```python
from build123d import *

# Parameters (mm, degrees)
F0_W     = 10
F0_H     = 45
F0_R     = 1.75
F1_DEPTH = 2
F2_W     = 4
F2_H     = 10
F3_DEPTH = 10
F4_R     = 3
F5_R     = 2.5
F6_DEPTH = 25.4


with BuildPart() as f1:
    # F0 (on Top) → F1 (new body)
    with BuildSketch(Plane.XY):
        with Locations((5, 22.5)):
            Rectangle(F0_W, F0_H)
        with Locations((5, 42.5)):
            Circle(F0_R, mode=Mode.SUBTRACT)
    extrude(amount=F1_DEPTH)

    # F2 (on face) → F3 (join)
    with BuildSketch(Plane.XY.offset(2)):
        with Locations((2, 5)):
            Rectangle(F2_W, F2_H)
    extrude(amount=F3_DEPTH)

    # F4
    f4_edges = [f1.edges().sort_by_distance(p)[0] for p in [
        (10, 45, 1),
        (10, 0, 1),
        (0, 45, 1),
        (2, 0, 12),
        (2, 10, 12),
    ]]
    fillet(f4_edges, radius=F4_R)

    # F5 (on face) → F6 (cut)
    with BuildSketch(Plane.YZ.offset(4)):
        with Locations((5, 8)):
            Circle(F5_R)
    extrude(amount=-F6_DEPTH, mode=Mode.SUBTRACT)


solid = f1.part
```
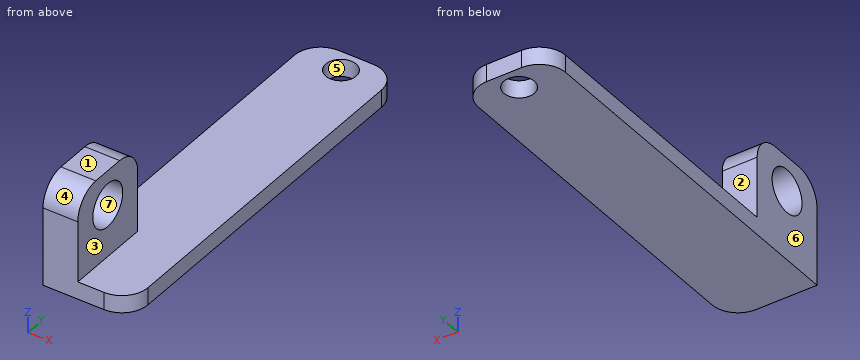
Work out the finished part from the listing and answer in its coordinate system (mm). Face numbers are marked on the shaded views. A direction names the side the tool comes from. Round coordinates to 2 decimals unless told otherwise and drop trailing zeros. Order: outer loops, then holes, each group sorted by start corner. A loop starts at its lowest first (then second) coordinate and runs counter-clockwise, first axis right, second up.
Q1. A cutting plane is placed at D-D, the plane z = 4. Determine the outline of the cut face in (x, y).
Solution:
outline: (0, 0) - (4, 0) - (4, 10) - (0, 10) - close
Q2. A cutting plane is placed at A-A, the plane y = 5. Determine the outline of the cut face in (x, z).
Solution:
outline: (0, 0) - (10, 0) - (10, 2) - (4, 2) - (4, 5.5) - (0, 5.5) - close; (0, 10.5) - (4, 10.5) - (4, 12) - (0, 12) - close
Q3. The mould has two halves that part along Y. Classify the marked faces 4, 5, 6 and 7: pulls with the +Y half, pulls with the -Y half, needs draft (parallel to the pull), parting line crosses it, or undercut.
Solution:
face 4: pulls with the -Y half
face 5: undercut
face 6: needs draft
face 7: undercut
Q4. A tool of negligible diameter and unlimited length cuts with its end or side. For the marked faces 1, 2 and 3, from which of +Z, -Z, +X, -X, +Y, -Y can it reach the whole face along a straight path? Write none if from no direction.
Solution:
face 1: +Z, +X, -X, +Y, -Y
face 2: +Z, +X, -X, +Y
face 3: +Z, +X, +Y, -Y
Q5. A cutting plane is placed at B-B, the plane z = 9.75. Determine the outline of the cut face in (x, y), then the cut area to 3 significant figures.
Solution:
outline: (0, 0.1) - (4, 0.1) - (4, 3.21) - (0, 3.21) - close; (0, 6.79) - (4, 6.79) - (4, 9.9) - (0, 9.9) - close
area: 25.0 mm2
Q6. Find the intervals of material crossed by line 1 along Z through (x, y) = (2, 5); line 2 along Z through (x, y) = (9.5, 35.5); line 3 along Y through (x, z) = (3.75, 8.5), in increasing order.
Solution:
line 1: z = 0 to 5.5, 10.5 to 12
line 2: z = 0 to 2
line 3: y = 0 to 2.55, 7.45 to 10
Q7. A cutting plane is placed at C-C, the plane x = 5. Determine the outline of the cut face in (y, z).
Solution:
outline: (0, 0) - (40.75, 0) - (40.75, 2) - (0, 2) - close; (44.25, 0) - (45, 0) - (45, 2) - (44.25, 2) - close
Q8. Given pin 1 Ø3 at (y, z) = (3.5, 6.5) entering from +X; pin 2 Ø5 at (x, y) = (4, 14.5) entering from +Z; pin 3 Ø4.5 at (x, z) = (2, 5) entering from +Y, each flat-ended and moving along its own axis, determine where each tip first touches the part or whether it passes through.
Solution:
pin 1: stops at x = 4
pin 2: stops at z = 2
pin 3: stops at y = 10
